Source: CAD feature listing. Evaluate the final solid. Frame: model axes, mm. A direction names the side the tool comes from. Give positions to 0.01 mm unless a question says otherwise; leave off trailing zeros. Order: outer loops, then holes, each group sorted by start corner. A loop starts at its lowest first (then second) coordinate and runs counter-clockwise, first axis right, second up. Notation, with made-up numbers: (78.5, -7) - (96.5, -7) arc R9 cw to (96.5, 2) - close; hole circle Ø11 at (43, -22.5). An arc over 180 degrees is marked (long way). Write each question's results on one line, items separated by ' | '. Start each with the question number.
Item 1: Section A-A on z = -5.5. Output: boundary loops of the cut face in (x, y).
Item 2: Mould query, pull axis Y, two halves, no side actions, for faces 6 (the cylindrical face through (-48.54, 27.55, -15.95)), 7 (the flat face through (-25, 30, -16)), 8 (the flat face through (38, 62, 0)), 9 (the flat face through (-25, 0, -16)). Classes: released by +Y, released by -Y, zero draft, split by the parting line, or undercut.
Item 3: Contact query for flat-ended pins moving along their axis: pin 1 Ø2 at (y, z) = (65.5, -6.5) entering from +X; pin 2 Ø8 at (x, z) = (-2.5, -22) entering from +Y; pin 3 Ø1 at (y, z) = (141, -4) entering from -X. Output: stop coordinate, or through.
Item 4: Section D-D on y = 90.5. Output: boundary loops of the cut face in (x, z).
Item 5: Line query: line 1 along Y through (x, z) = (-36.5, -24); line 2 along X through (y, z) = (9, -24); line 3 along Z through (x, y) = (51, 70). Output: solid intervals per line, ascending.
Item 6: Section B-B on x = 6. Output: boundary loops of the cut face in (y, z), and give its area (3 significant figures).
Item 7: Section C-C on z = -29.5. Output: boundary loops of the cut face in (x, y).
Item 8: Set-up query: faces 1 (the flat face through (-26, 25, -16)), 2 (the flat face through (0, 15, -16)), 3 (the flat face through (113.673, 140, -4)), 4 (the flat face through (-19.2, 25.2, -32.36)), 5 (the cylindrical face through (0.644, 20.735, -3.974)). Return all of +Z, -Z, +X, -X, +Y, -Y with unobstructed straight access to the full face (end or side cutting, diameter ignored); none if empty.
```python
from build123d import *

# Parameters (mm, degrees)
EXTRUDE001_DEPTH = 32.36
EXTRUDE_DEPTH    = 8.06


with BuildPart() as extrude001:
    # Sketch001 → Extrude001 (new body)
    with BuildSketch(Plane.XY):
        with BuildLine():
            Line((-46.04, 25), (-5, 25))
            Line((-5, 25), (-5, 5))
            Line((-5, 5), (-46.04, 5))
            ThreePointArc((-46.04, 5), (-48.54, 2.5), (-46.04, 0))
            Line((-46.04, 0), (-2.5, 0))
            ThreePointArc((-2.5, 0), (-0.732233, 0.732233), (0, 2.5))
            Line((0, 27.5), (0, 2.5))
            ThreePointArc((0, 27.5), (-0.732233, 29.267767), (-2.5, 30))
            Line((-46.04, 30), (-2.5, 30))
            ThreePointArc((-46.04, 30), (-48.54, 27.5), (-46.04, 25))
        make_face()
    extrude(amount=-EXTRUDE001_DEPTH)


with BuildPart() as fusion:
    # Sketch → Extrude (new body)
    with BuildSketch(Plane.XY):
        with BuildLine():
            Line((-46.04, 25), (-5, 25))
            Line((-5, 25), (-5, 5))
            Line((-5, 5), (-46.04, 5))
            ThreePointArc((-46.04, 5), (-48.54, 2.5), (-46.04, 0))
            Line((-46.04, 0), (-2.5, 0))
            ThreePointArc((-2.5, 0), (-0.732233, 0.732233), (0, 2.5))
            Line((0, 17.715099), (0, 2.5))
            ThreePointArc((2.400936, 23.171642), (0.626774, 20.695802), (0, 17.715099))
            Line((2.400936, 23.171642), (125, 135.512986))
            ThreePointArc((125, 135.512986), (125.478432, 136.180638), (125.647452, 136.984434))
            Line((125.647452, 136.984434), (125.647452, 141.966204))
            ThreePointArc((125.647452, 141.966204), (123.651667, 143.96199), (121.655881, 141.966204))
            Line((121.655881, 141.966204), (121.655881, 139.903136))
            ThreePointArc((117.664309, 139.903136), (119.660095, 137.90735), (121.655881, 139.903136))
            Line((117.664309, 139.903136), (117.664309, 141.966204))
            ThreePointArc((117.664309, 141.966204), (115.668524, 143.96199), (113.672738, 141.966204))
            Line((113.672738, 141.966204), (113.672738, 136.984434))
            ThreePointArc((113.025285, 135.512986), (113.503718, 136.180638), (113.672738, 136.984434))
            Line((0, 31.944394), (113.025285, 135.512986))
            ThreePointArc((-5, 30), (-2.317619, 30.503205), (0, 31.944394))
            Line((-46.04, 30), (-5, 30))
            ThreePointArc((-46.04, 30), (-48.54, 27.5), (-46.04, 25))
        make_face()
    extrude(amount=-EXTRUDE_DEPTH)

    # Fusion: union Extrude001
    add(extrude001.part)


solid = fusion.part
```
Evaluation:
1) outline: (-46.04, 0) - (-2.5, 0) arc R2.5 ccw to (0, 2.5) - (0, 17.72) arc R7.4 cw to (2.4, 23.17) - (125, 135.51) arc R2 ccw to (125.65, 136.98) - (125.65, 141.97) arc R2 ccw to (121.66, 141.97) - (121.66, 139.9) arc R2 cw to (117.66, 139.9) - (117.66, 141.97) arc R2 ccw to (113.67, 141.97) - (113.67, 136.98) arc R2 cw to (113.03, 135.51) - (0, 31.94) arc R7.4 cw to (-5, 30) - (-46.04, 30) arc R2.5 ccw to (-46.04, 25) - (-5, 25) - (-5, 5) - (-46.04, 5) arc R2.5 ccw to start
2) face 6: undercut | face 7: released by +Y | face 8: zero draft | face 9: released by -Y
3) pin 1: stops at x = 49.69 | pin 2: stops at y = 30 | pin 3: stops at x = 113.67
4) outline: (63.9, -8.06) - (75.88, -8.06) - (75.88, 0) - (63.9, 0) - close
5) line 1: y = 0 to 5, 25 to 30 | line 2: x = -5 to 0 | line 3: z = -8.06 to 0
6) outline: (26.47, -8.06) - (37.44, -8.06) - (37.44, 0) - (26.47, 0) - close | area: 88.4 mm^2
7) outline: (-46.04, 0) - (-2.5, 0) arc R2.5 ccw to (0, 2.5) - (0, 27.5) arc R2.5 ccw to (-2.5, 30) - (-46.04, 30) arc R2.5 ccw to (-46.04, 25) - (-5, 25) - (-5, 5) - (-46.04, 5) arc R2.5 ccw to start
8) face 1: +Z, -Z, -X | face 2: -Z, +X, -Y | face 3: +Z, -Z, -X, +Y | face 4: -Z, +X, -X, +Y, -Y | face 5: +Z, -Z, +X, -Y
